Part print with two shaded views. Sizes in mm from the minimum x, y, z corner. A direction names the side the tool comes from. Coordinates: 2 decimals unless noted, no trailing zeros. Write each loop counter-clockwise with the first axis right and the second up, starting at its lowest first coordinate (ties: lowest second). Pieces come first, ordered by that corner, then holes.
Q1. Band-saw the part on B-B, the plane z = 3.75. Write the cut outline in (x, y) (1 decimal).
Q2. Pull direction X, two halves, no side cores. Call the marked faces 4, 5 and 6: released by +X, released by -X, zero draft, split by the parting line, or undercut.
Q3. Drill centre lines: probe 1 along Y at (x, z) = (17.78, 0.2) (1 decimal); probe 2 along X at (y, z) = (14, 6.25); probe 3 along X at (y, z) = (40, 4) (1 decimal). Where is each one in solid material? Low to high.
Q4. Band-saw the part on A-A, the plane x = 17.78. Write the cut outline in (y, z) (1 decimal).
Q5. Band-saw the part on C-C, the plane y = 47. Write the cut outline in (x, z) (1 decimal).
Q6. Which spindle directions (+Z, -Z, +X, -X, +Y, -Y) get a long thin tool onto all of the face, cutting with end or side? Do the marked faces 1, 2 and 3. Say none if no direction does.
Q7. Pin check, flat tips, straight feed: P1, Ø1.9, axis at x = 17.78, y = 4.445, coming from the -Z side; P2, Ø5.5, axis at x = 14.5, y = 7, coming from the +Z side; P3, Ø1.4, axis at x = 33.5, y = 24.5, coming from the +Z side (1 decimal). Stop position of each tip, or through.
Q8. Band-saw the part on D-D, the plane x = 4. Write the cut outline in (y, z).
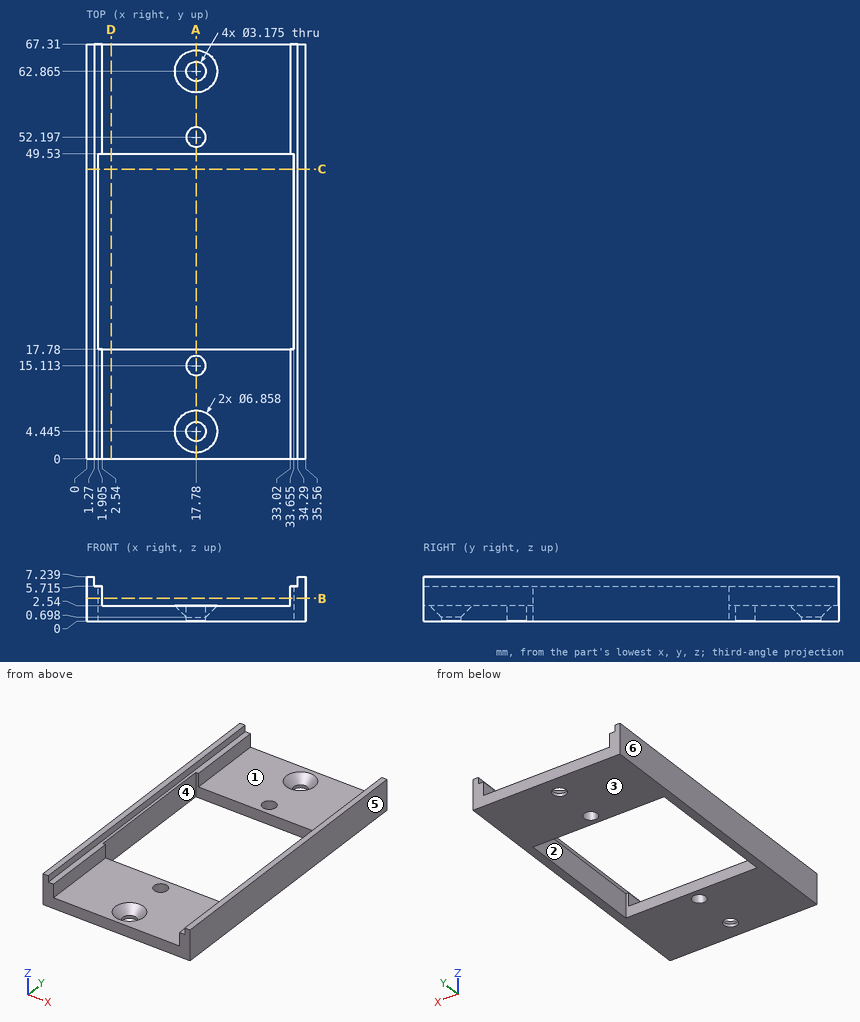
Answer sheet:
1. outline: (0, 0) - (2.5, 0) - (2.5, 17.8) - (1.9, 17.8) - (1.9, 49.5) - (2.5, 49.5) - (2.5, 67.3) - (0, 67.3) - close; (33, 0) - (35.6, 0) - (35.6, 67.3) - (33, 67.3) - (33, 49.5) - (33.7, 49.5) - (33.7, 17.8) - (33, 17.8) - close
2. face 4: undercut
2. face 5: released by +X
2. face 6: released by -X
3. probe 1: y = 0 to 2.9, 6 to 13.5, 16.7 to 17.8, 49.5 to 50.6, 53.8 to 61.3, 64.5 to 67.3
3. probe 2: x = 0 to 1.27, 34.29 to 35.56
3. probe 3: x = 0 to 1.9, 33.7 to 35.6
4. outline: (0, 0) - (2.9, 0) - (2.9, 0.7) - (1, 2.5) - (0, 2.5) - close; (6, 0) - (13.5, 0) - (13.5, 2.5) - (7.9, 2.5) - (6, 0.7) - close; (16.7, 0) - (17.8, 0) - (17.8, 2.5) - (16.7, 2.5) - close; (49.5, 0) - (50.6, 0) - (50.6, 2.5) - (49.5, 2.5) - close; (53.8, 0) - (61.3, 0) - (61.3, 0.7) - (59.4, 2.5) - (53.8, 2.5) - close; (64.5, 0) - (67.3, 0) - (67.3, 2.5) - (66.3, 2.5) - (64.5, 0.7) - close
5. outline: (0, 0) - (1.9, 0) - (1.9, 5.7) - (1.3, 5.7) - (1.3, 7.2) - (0, 7.2) - close; (33.7, 0) - (35.6, 0) - (35.6, 7.2) - (34.3, 7.2) - (34.3, 5.7) - (33.7, 5.7) - close
6. face 1: +Z, +Y, -Y
6. face 2: +Z, -Z
6. face 3: -Z, +X, -X, +Y, -Y
7. P1: passes through
7. P2: stops at z = 2.54
7. P3: stops at z = 5.7
8. outline: (0, 0) - (17.78, 0) - (17.78, 2.54) - (0, 2.54) - close; (49.53, 0) - (67.31, 0) - (67.31, 2.54) - (49.53, 2.54) - close
